Check sheet for the modelled part. Datum: model origin and axes. Units: mm. A direction names the side the tool comes from. Give positions to 0.01 mm unless a question says otherwise; leave off trailing zeros. Write each loop counter-clockwise with the first axis right and the second up, starting at its lowest first coordinate (ties: lowest second). Pieces come first, ordered by that corner, then holes. Notation, with made-up numbers: (68.5, -26) -> (95.5, -26) arc R24 cw to (95.5, 5) -> close; hole circle Ø7 at (-35, -4.5). An arc over 180 degrees is marked (long way). Answer as a JSON object with one key per item and string values.
Autodesk Fusion 360 part; units mm, degrees
sketch "Sketch1" plane through (0, 0, 0) normal (1, 0, 0) x (0, 1, 0)
  line L0 (0, 0) -> (0, 5.5344)
  line L1 (0, 5.5344) -> (63.2584, 0)
  line L2 (63.2584, 0) -> (63.8118, 6.3258)
  line L3 (63.8118, 6.3258) -> (61.2815, 6.5472) construction
  line L4 (61.2815, 6.5472) -> (60.728, 0.2214) construction
  line L5 (0, 0) -> (63.2584, 0) construction
  line L6 (63.2584, 0) -> (63.2584, -1.905) construction
  line L7 (63.2584, -1.905) -> (0, -1.905)
  line L8 (0, -1.905) -> (0, 0)
  line L9 (66.3421, 6.1045) -> (65.7887, -0.2214)
  line L10 (63.8118, 6.3258) -> (66.3421, 6.1045) construction
  line L11 (63.2584, 0) -> (65.8081, 0) construction
  line L12 (65.8081, 0) -> (65.8081, -1.905)
  line L13 (65.8081, -1.905) -> (63.2584, -1.905)
  line L14 (63.8118, 6.3258) -> (66.3421, 6.1045) construction
  line L15 (63.8118, 6.3258) -> (66.3421, 6.3258)
  line L16 (66.3421, 6.3258) -> (66.3421, 6.1045)
  dimension "d1" = 2.54
  dimension "d3" = 6.35
  dimension "d4" = 63.5
  dimension "d7" = 1.905
  dimension "d15" = 5
extrude "Extrude1" add sketch "Sketch1" along normal blind 135.255
sketch "Sketch2" plane through (135.255, 0, 0) normal (1, 0, 0) x (0, 1, 0)
  line L0 (65.8081, -1.905) -> (65.8081, 0)
  line L1 (65.8081, 0) -> (66.3421, 6.1045)
  line L2 (63.8118, 6.3258) -> (63.2584, 0)
  line L3 (63.2584, 0) -> (0, 5.5344)
  line L4 (0, 5.5344) -> (0, -1.905)
  line L5 (0, -1.905) -> (65.8081, -1.905)
  line L6 (63.8118, 6.3258) -> (0, 5.5344)
  line L7 (63.8118, 6.3258) -> (66.3421, 6.3572)
  line L8 (66.3421, 6.3572) -> (66.3421, 6.1045)
  line L9 (66.3421, 6.3258) -> (63.8118, 6.3258)
  line L10 (66.3421, 6.1045) -> (66.3421, 6.3258)
extrude "Extrude2" add sketch "Sketch2" along normal blind 1.27 contours L0 L1 L2 L3 L4 L5 L8 L9 L10 | L2 L3 L6
extrude "Extrude3" add 1 faces at (136.525, 43.2066, 0.8386) along direction (-1, 0, 0) blind 1.27 from surface at 136.525
fillet "Fillet1" radius 1.27 8 edges at (0, 63.5351, 3.1629) (135.255, 63.5351, 3.1629) (-1.27, 66.0751, 3.0522) (-1.27, 65.8081, -0.9525) (136.525, 66.0751, 3.0522) (136.525, 65.8081, -0.9525) (-1.27, 0, 1.8147) (136.525, 0, 1.8147)
1. Go/stop test with flat-tipped pins: P1, Ø5, axis at x = 43, y = 11, coming from the +Z side; P2, Ø1, axis at x = 81.5, z = 1.5, coming from the -Y side; P3, Ø4, axis at x = 103, z = 3, coming from the +Y side; P4, Ø5, axis at x = 17.5, y = 30, coming from the +Z side. Record where each tip stops, or that it passes through.
Determined:
{"P1": "z = 4.79", "P2": "y = 0", "P3": "y = 66.25", "P4": "z = 3.13"}
2. Access from +Z, -Z, +X, -X, +Y, -Y to the whole of each face (thin tool, end or side, straight path). Record for faces 4 (the face through (-1.27, 33, 2)), 5 (the face through (66.681, 31.186, 2.806)).
Determined:
{"face 4": "+Z, -Z, -X, +Y, -Y", "face 5": "+Z"}
3. Mould release check, pull along Y, two halves, no side actions. Record for faces 1 (the face through (66.7, 63.53, 3.12)), 2 (the face through (136.525, 33, 2)), 3 (the face through (69, 0, 2)): released by +Y, released by -Y, zero draft, split by the parting line, or undercut.
Determined:
{"face 1": "undercut", "face 2": "zero draft", "face 3": "released by -Y"}
4. Scan lines: L1, parallel to X at y = 50, z = 3.75 (3 decimals); L2, parallel to Y at x = 25, z = -1; L3, parallel to Z at x = 72.5, y = 8.5 (3 decimals). Record each from-to range of solid material in increasing order. Write a range as [from, to].
Determined:
{"L1": "[-1.27, 0], [135.255, 136.525]", "L2": "[0, 65.81]", "L3": "[-1.905, 4.791]"}
5. Sectioned sample at B-B, the plane y = 22. Enter the section's corners in (x, z) (3 decimals), plus the area to 3 significant figures.
Determined:
{"outline": "(-1.27, -1.905) -> (136.525, -1.905) -> (136.525, 5.807) -> (135.255, 5.807) -> (135.255, 3.61) -> (0, 3.61) -> (0, 5.807) -> (-1.27, 5.807) -> close", "area": "765 mm^2"}
